Work out the finished part from the listing and answer in its coordinate system (mm). A direction names the side the tool comes from. Give positions to 0.01 mm unless a question says otherwise; leave off trailing zeros. Order: outer loops, then holes, each group sorted by start corner. A loop starts at its lowest first (then second) coordinate and runs counter-clockwise, first axis right, second up. Notation, with made-up numbers: (75, -39) - (91, -39) arc R5 ccw to (91, -35) - close; hole circle Ø8 at (54.25, -22). An arc over 180 degrees is marked (long way). Put each result on its own line as item: value.
```python
from build123d import *

# Parameters (mm, degrees)
F0_W      = 91.44
F0_H      = 66.04
F0_W_2    = 86.36
F0_H_2    = 60.96
F1_DEPTH  = 25.4
F0_W_3    = 101.6
F0_H_3    = 76.2
F2_DEPTH  = 76.2
F3_W      = 2.54
F3_H      = 38.1
F4_DEPTH  = 5.08
F5_DEPTH  = 5.08
F6_W      = 2.54
F6_H      = 38.1
F7_DEPTH  = 5.08
F8_W      = 71.12
F8_H      = 10.16
F9_DEPTH  = 15.24
F10_W     = 71.12
F10_H     = 10.16
F11_DEPTH = 15.24
F12_W     = 10.16
F12_H     = 66.04
F13_DEPTH = 7.62


with BuildPart() as f1:
    # F0 (on Top) → F1 (new body)
    with BuildSketch(Plane.XY):
        Rectangle(F0_W, F0_H)
        Rectangle(F0_W_2, F0_H_2, mode=Mode.SUBTRACT)
    extrude(amount=F1_DEPTH)

    # F0 (on Top) → F2 (join)
    with BuildSketch(Plane.XY):
        Rectangle(F0_W_3, F0_H_3)
        Rectangle(F0_W, F0_H, mode=Mode.SUBTRACT)
    extrude(amount=F2_DEPTH)

    # F3 (on face) → F4 (cut)
    with BuildSketch(Plane.YZ.offset(50.8)):
        with Locations((-29.21, 44.45)):
            Rectangle(F3_W, F3_H)
        with Locations((-24.13, 44.45)):
            Rectangle(F3_W, F3_H)
        with Locations((-19.05, 44.45)):
            Rectangle(F3_W, F3_H)
        with Locations((-13.97, 44.45)):
            Rectangle(F3_W, F3_H)
        with Locations((-8.89, 44.45)):
            Rectangle(F3_W, F3_H)
        with Locations((-3.81, 44.45)):
            Rectangle(F3_W, F3_H)
        with Locations((3.81, 44.45)):
            Rectangle(F3_W, F3_H)
        with Locations((8.89, 44.45)):
            Rectangle(F3_W, F3_H)
        with Locations((13.97, 44.45)):
            Rectangle(F3_W, F3_H)
        with Locations((19.05, 44.45)):
            Rectangle(F3_W, F3_H)
        with Locations((24.13, 44.45)):
            Rectangle(F3_W, F3_H)
        with Locations((29.21, 44.45)):
            Rectangle(F3_W, F3_H)
    extrude(amount=-F4_DEPTH, mode=Mode.SUBTRACT)

    # F0 (on Top) → F5 (join)
    with BuildSketch(Plane.XY):
        Rectangle(F0_W_2, F0_H_2)
    extrude(amount=F5_DEPTH)

    # F6 (on face) → F7 (cut)
    with BuildSketch(Plane(origin=(-50.8, 0, 0), x_dir=(0, -1, 0), z_dir=(-1, 0, 0))):
        with Locations((-3.81, 44.45)):
            Rectangle(F6_W, F6_H)
        with Locations((3.81, 44.45)):
            Rectangle(F6_W, F6_H)
        with Locations((8.89, 44.45)):
            Rectangle(F6_W, F6_H)
        with Locations((13.97, 44.45)):
            Rectangle(F6_W, F6_H)
        with Locations((-8.89, 44.45)):
            Rectangle(F6_W, F6_H)
        with Locations((-13.97, 44.45)):
            Rectangle(F6_W, F6_H)
        with Locations((19.05, 44.45)):
            Rectangle(F6_W, F6_H)
        with Locations((24.13, 44.45)):
            Rectangle(F6_W, F6_H)
        with Locations((29.21, 44.45)):
            Rectangle(F6_W, F6_H)
        with Locations((-19.05, 44.45)):
            Rectangle(F6_W, F6_H)
        with Locations((-24.13, 44.45)):
            Rectangle(F6_W, F6_H)
        with Locations((-29.21, 44.45)):
            Rectangle(F6_W, F6_H)
    extrude(amount=-F7_DEPTH, mode=Mode.SUBTRACT)

    # F8 (on face) → F9 (join)
    with BuildSketch(Plane(origin=(-50.8, 0, 0), x_dir=(0, -1, 0), z_dir=(-1, 0, 0))):
        with Locations((0, 71.12)):
            Rectangle(F8_W, F8_H)
    extrude(amount=F9_DEPTH)

    # F10 (on face) → F11 (join)
    with BuildSketch(Plane.YZ.offset(50.8)):
        with Locations((0, 71.12)):
            Rectangle(F10_W, F10_H)
    extrude(amount=F11_DEPTH)

    # F12 (on face) → F13 (cut)
    with BuildSketch(Plane(origin=(0, 0, 66.04), x_dir=(1, 0, 0), z_dir=(0, 0, -1))):
        with Locations((58.42, 0)):
            Rectangle(F12_W, F12_H)
        with Locations((-58.42, 0)):
            Rectangle(F12_W, F12_H)
    extrude(amount=-F13_DEPTH, mode=Mode.SUBTRACT)


solid = f1.part
```
(1) Section A-A, the plane z = 23.5 is taken. Write down the section's boundary in (x, y), then the cut area to 3 significant figures.
Geometry check:
outline: (-50.8, -38.1) - (50.8, -38.1) - (50.8, 38.1) - (-50.8, 38.1) - close; hole (-43.18, -30.48) - (43.18, -30.48) - (43.18, 30.48) - (-43.18, 30.48) - close
area: 2,480 mm²
(2) Straight lines are drawn through the part: line 1 (X direction, y = 32.5, z = 67.5); line 2 (Y direction, x = 11.5, z = 62.5); line 3 (X direction, y = -11.5, z = 50.5). For each, find the intervals that lie inside material, in ascending order.
Geometry check:
line 1: x = -66.04 to -63.5, -53.34 to -45.72, 45.72 to 53.34, 63.5 to 66.04
line 2: y = -38.1 to -33.02, 33.02 to 38.1
line 3: x = -50.8 to -45.72, 45.72 to 50.8
(3) A tool of negligible diameter and unlimited length cuts with its end or side. For faces 1 (the face through (58, 33.02, 70)), 2 (the face through (48, -5.08, 44)), 3 (the face through (-1, -33.02, 50)), from which of +Z, -Z, +X, -X, +Y, -Y can it reach the whole face along a straight path? Write none if from no direction.
Geometry check:
face 1: -Z
face 2: +X, -X
face 3: +Z
(4) Section D-D, the plane z = 40.5 is taken. Count the separate pieces of the cut face and the enclosed holes in it, then the cut area to 3 significant figures.
Geometry check:
separate pieces: 24
enclosed holes: 0
area: 1,390 mm²
(5) Determine the mould class of faces 4 (the face through (48, 27.94, 44)), 5 (the face through (58, 35.56, 71)), 6 (the face through (-1, 1, 0)) for opening direction Z: pulls with the +Z half, pulls with the -Z half, needs draft (parallel to the pull), parting line crosses it, or undercut.
Geometry check:
face 4: undercut
face 5: needs draft
face 6: pulls with the -Z half
(6) Given pin 1 (16.5 mm diameter, centred on y = 12, z = 20, fed in from +X); pin 2 (10 mm diameter, centred on y = 27, z = 12, fed in from -X); pin 3 (4.5 mm diameter, centred on x = -60.5, y = 13, fed in from -Z), each flat-ended and moving along its own axis, determine where each tip first touches the part or whether it passes through.
Geometry check:
pin 1: stops at x = 50.8
pin 2: stops at x = -50.8
pin 3: stops at z = 73.66
(7) Section B-B, the plane x = 56.5 is taken. Write down the section's boundary in (y, z), then the cut area to 3 significant figures.
Geometry check:
outline: (-35.56, 66.04) - (-33.02, 66.04) - (-33.02, 73.66) - (33.02, 73.66) - (33.02, 66.04) - (35.56, 66.04) - (35.56, 76.2) - (-35.56, 76.2) - close
area: 219 mm²
(8) Section C-C, the plane z = 70.5 is taken. Write down the section's boundary in (x, y).
Geometry check:
outline: (-66.04, -35.56) - (-50.8, -35.56) - (-50.8, -38.1) - (50.8, -38.1) - (50.8, -35.56) - (66.04, -35.56) - (66.04, 35.56) - (50.8, 35.56) - (50.8, 38.1) - (-50.8, 38.1) - (-50.8, 35.56) - (-66.04, 35.56) - close; hole (-63.5, -33.02) - (-53.34, -33.02) - (-53.34, 33.02) - (-63.5, 33.02) - close; hole (-45.72, -33.02) - (45.72, -33.02) - (45.72, 33.02) - (-45.72, 33.02) - close; hole (53.34, -33.02) - (63.5, -33.02) - (63.5, 33.02) - (53.34, 33.02) - close
